Part model, mm, in its own coordinate system. Face numbers are marked on the shaded views. A direction names the side the tool comes from. Round coordinates to 2 decimals unless told otherwise and drop trailing zeros. Loops run counter-clockwise (first coordinate to the right, second up) from the corner with the lowest first, then second, coordinate; pieces in that order, holes last.
1) Band-saw the part on C-C, the plane x = 5.5. Write the cut outline in (y, z), then the cut area to 3 significant figures.
2) Band-saw the part on B-B, the plane y = 2. Write the cut outline in (x, z), then the cut area to 3 significant figures.
3) 3-axis set-ups, long thin cutter, end or side, ignore diameter. For the marked faces 1 and 2: which of +Z, -Z, +X, -X, +Y, -Y reach the whole face in a straight line?
4) Drop flat-ended pins along their axis: P1, Ø10, axis at y = 1.5, z = -65.5, coming from the -X side; P2, Ø12, axis at x = 11, z = 103.5, coming from the +Y side. Give the stop position or say it passes through.
5) Band-saw the part on A-A, the plane z = -212.5. Write the cut outline in (x, y) (3 decimals).
6) Probe line 1 (X direction, y = -11, z = -25.5); line 2 (Y direction, x = 8, z = 129); line 3 (Y direction, x = 14.5, z = -234.5). List the from-to ranges inside material, lowest first.
from build123d import *

# Parameters (mm, degrees)
BOSS_EXTRUDE1_DEPTH = 304.8
SKETCH3_W           = 30.020943331
SKETCH3_H           = 21.596699029
CUT_EXTRUDE1_DEPTH  = 612.317372565


with BuildPart() as part:
    # Sketch2 → Boss-Extrude1 (new, symmetric)
    with BuildSketch(Plane.XY):
        with BuildLine():
            Line((-25.4, -38.1), (25.4, -38.1))
            Line((25.4, -38.1), (25.4, 38.1))
            Line((25.4, 38.1), (22.225, 38.1))
            ThreePointArc((22.225, 38.1), (19.97993597, 37.17006403), (19.05, 34.925))
            Line((19.05, 34.925), (19.05, -26.9748))
            ThreePointArc((19.05, -26.9748), (17.651376302, -30.351376302), (14.2748, -31.75))
            Line((14.2748, -31.75), (-22.225, -31.75))
            ThreePointArc((-22.225, -31.75), (-24.47006403, -32.67993597), (-25.4, -34.925))
            Line((-25.4, -34.925), (-25.4, -38.1))
        make_face()
    extrude(amount=BOSS_EXTRUDE1_DEPTH, both=True)

    # Sketch3 → Cut-Extrude1 (cut, through all)
    with BuildSketch(Plane.XY.offset(304.8)):
        with Locations((23.779344144, 30.05923535)):
            Rectangle(SKETCH3_W, SKETCH3_H)
    extrude(amount=-CUT_EXTRUDE1_DEPTH, mode=Mode.SUBTRACT)


solid = part.part
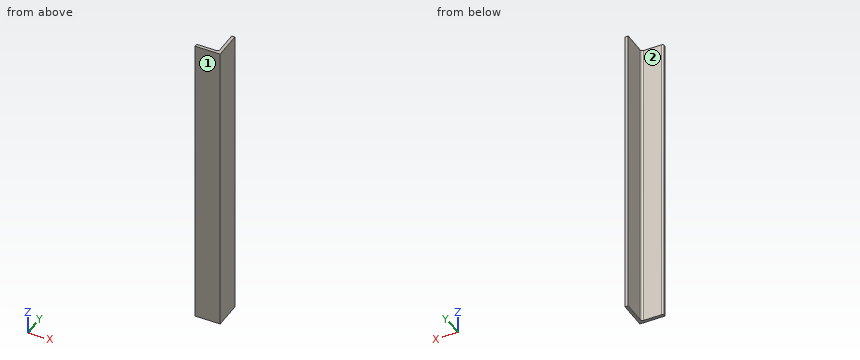
Reported:
1. outline: (-38.1, -304.8) - (-31.75, -304.8) - (-31.75, 304.8) - (-38.1, 304.8) - close
1. area: 3,870 mm2
2. outline: (19.05, -304.8) - (25.4, -304.8) - (25.4, 304.8) - (19.05, 304.8) - close
2. area: 3,870 mm2
3. face 1: +Z, -Z, +X, -X, -Y
3. face 2: +Z, -Z, -X, +Y
4. P1: stops at x = 19.05
4. P2: stops at y = -30.9
5. outline: (-25.4, -38.1) - (25.4, -38.1) - (25.4, 19.261) - (19.05, 19.261) - (19.05, -26.975) arc R4.775 cw to (14.275, -31.75) - (-22.225, -31.75) arc R3.175 ccw to (-25.4, -34.925) - close
6. line 1: x = 19.05 to 25.4
6. line 2: y = -38.1 to -31.75
6. line 3: y = -38.1 to -31.74
